The model under review builds one solid part; all positions refer to its coordinate system, in mm. A direction names the side the tool comes from. Coordinates: 2 decimals unless noted, no trailing zeros. Write each loop counter-clockwise with the first axis right and the second up, starting at its lowest first coordinate (ties: lowest second). Pieces come first, ordered by that corner, then holes.
1) Mouldability with a two-part tool opening along Z and no side actions: class faces 3 (the flat face through (5.4, -15.1, -30.48)), 4 (the cylindrical face through (-14.61, 11.21, 19.14)), 5 (the flat face through (0, 0, 203.2)), 6 (the flat face through (-5.4, -15.1, 27.94)) as released by +Z, released by -Z, zero draft, split by the parting line, or undercut.
2) For line 1 (Y direction, x = -1, z = -183); line 2 (X direction, y = 14.5, z = 167); line 3 (X direction, y = -4, z = -26), list the stretches that pass through material, from the lowest coordinate up.
3) Machinability: for faces 1 (the conical face through (-2.831, 12.747, -202.581)), 2 (the flat face through (-5.4, -15.1, -27.94)), which of the approach directions +Z, -Z, +X, -X, +Y, -Y give a long, thin tool a straight path to every point of the face, cutting with its end or side? Answer none if there is none.
4) For P1, Ø12, axis at x = -11.5, y = -9.5, coming from the +Z side; P2, Ø1.5, axis at y = -12, z = 156.5, coming from the -X side; P3, Ø3, axis at x = -11.5, z = 140.5, coming from the -Y side; P4, Ø4, axis at x = -6, z = -23.5, coming from the -Y side, all flat-tipped, find the tip position at first contact; note any pin that passes through.
5) Add section A-A, the plane z = -39.5. State the section outline as (x, y) points (3 decimals), then the cut area to 3 significant figures.
from build123d import *


with BuildPart() as f1:
    # F0 (on Front) → F1 (revolve)
    with BuildSketch(Plane.XZ):
        with BuildLine():
            Line((12.7, 203.2), (0, 203.2))
            Line((0, 203.2), (0, -203.2))
            Line((0, -203.2), (12.7, -203.2))
            Line((12.7, -203.2), (18.415, -193.30133))
            Line((18.415, -193.30133), (18.415, -180.60133))
            Line((18.415, -180.60133), (15.875, -180.60133))
            Line((15.875, -180.60133), (15.875, -178.06133))
            Line((15.875, -178.06133), (18.415, -178.06133))
            Line((18.415, -178.06133), (18.415, -30.48))
            Line((18.415, -30.48), (15.875, -30.48))
            Line((15.875, -30.48), (15.875, -27.94))
            Line((15.875, -27.94), (18.415, -27.94))
            Line((18.415, -27.94), (18.415, -12.7))
            ThreePointArc((18.415, -12.7), (13.564032, 0), (18.415, 12.7))
            Line((18.415, 12.7), (18.415, 25.4))
            Line((18.415, 25.4), (15.875, 25.4))
            Line((15.875, 25.4), (15.875, 27.94))
            Line((15.875, 27.94), (18.415, 27.94))
            Line((18.415, 27.94), (18.415, 166.63133))
            Line((18.415, 166.63133), (15.875, 166.63133))
            Line((15.875, 166.63133), (15.875, 169.17133))
            Line((15.875, 169.17133), (18.415, 169.17133))
            Line((18.415, 169.17133), (18.415, 181.87133))
            Line((18.415, 181.87133), (12.7, 203.2))
        make_face()
    revolve(axis=Axis((0, 0, 0), (0, 0, -1)))


solid = f1.part
Geometry results:
1. face 3: undercut
1. face 4: zero draft
1. face 5: released by +Z
1. face 6: undercut
2. line 1: y = -18.39 to 18.39
2. line 2: x = -6.46 to 6.46
2. line 3: x = -17.98 to 17.98
3. face 1: -Z
3. face 2: none
4. P1: stops at z = 203.2
4. P2: stops at x = -14.58
4. P3: stops at y = -15.46
4. P4: stops at y = -17.98
5. outline: circle Ø36.83 at (0, 0)
5. area: 1,070 mm2
